Autodesk Fusion 360 part; units mm, degrees
sketch "Sketch1" plane through (0, 0, 0) normal (0, 0, 1) x (1, 0, 0)
  line L0 (0, 0) -> (69, 0)
  line L1 (69, 0) -> (69, 140)
  line L2 (69, 140) -> (0, 140)
  line L3 (0, 140) -> (0, 0)
  line L4 (0, 140) -> (-3, 140)
  line L5 (-3, 140) -> (-3, 0)
  line L6 (-3, 0) -> (0, 0)
  line L7 (0, 0) -> (0, 140)
  line L8 (69, 140) -> (72, 140)
  line L9 (72, 140) -> (72, 0)
  line L10 (72, 0) -> (69, 0)
  line L11 (69, 0) -> (69, 140)
  line L12 (34.5, 140) -> (34.5, 0) construction
  line L13 (25, 0) -> (44, 0)
  line L14 (44, 0) -> (44, 2)
  line L15 (44, 2) -> (25, 2)
  line L16 (25, 2) -> (25, 0)
  line L17 (34.5, 2) -> (34.5, 0) construction
  line L18 (53.1198, 29) -> (65.1198, 29)
  line L19 (65.1198, 29) -> (65.1198, 15)
  line L20 (65.1198, 15) -> (53.1198, 15)
  line L21 (53.1198, 15) -> (53.1198, 29)
  circle A0 centre (8, 75) radius 3.175
  circle A1 centre (61.6198, 40) radius 3.5
  line L22 (65.1198, 29) -> (65.1198, 49) construction
  dimension "d1" = 140
  dimension "d3" = 3
  dimension "d4" = 3
  dimension "d30" = 75
  dimension "d31" = 2
  dimension "d32" = 19
  dimension "d33" = 14
  dimension "d34" = 12
  dimension "d35" = 6.35
  dimension "d36" = 65
  dimension "d37" = 7
  dimension "d38" = 40
  dimension "d39" = 15
extrude "Extrude1" add sketch "Sketch1" along normal blind 3 contours L0 L1 L2 L3 L7 L11 L14 L15 L16
extrude "Extrude2" add sketch "Sketch1" along normal blind 40 contours L3 L4 L5 L6 L7 | L1 L8 L9 L10 L11
sketch "Sketch3" plane through (72, 0, 0) normal (1, 0, 0) x (0, 1, 0)
  line L0 (0, 0) -> (140, 0)
  line L1 (140, 0) -> (140, 40)
  line L2 (140, 40) -> (0, 40)
  line L3 (0, 40) -> (0, 0)
  line L4 (140, 0) -> (0, 0)
  line L5 (70, 40) -> (70, 0) construction
  line L6 (17.5, 40) -> (22.5, 40)
  line L7 (22.5, 40) -> (22.5, 37)
  line L8 (20.5, 35) -> (19.5, 35)
  line L9 (17.5, 37) -> (17.5, 40)
  arc A0 (17.5, 37) -> (19.5, 35) centre (19.5, 37) ccw
  arc A1 (20.5, 35) -> (22.5, 37) centre (20.5, 37) ccw
  line L10 (20, 40) -> (20, 35) construction
  line L11 (117.5, 40) -> (122.5, 40)
  line L12 (122.5, 40) -> (122.5, 37)
  line L13 (120.5, 35) -> (119.5, 35)
  line L14 (117.5, 37) -> (117.5, 40)
  arc A2 (117.5, 37) -> (119.5, 35) centre (119.5, 37) ccw
  arc A3 (120.5, 35) -> (122.5, 37) centre (120.5, 37) ccw
  line L15 (120, 35) -> (120, 40) construction
  point P0 (17.5, 35)
  point P1 (117.5, 35)
  dimension "d18" = 5
  dimension "d19" = 5
  dimension "d20" = 2
  dimension "d21" = 2
  dimension "d23" = 5
  dimension "d24" = 2
  dimension "d25" = 2
  dimension "d26" = 5
  dimension "d27" = 100
extrude "Extrude3" cut sketch "Sketch3" along normal mid plane 200 contours L2 L6 L7 L8 L9 A0 A1 | L2 L11 L12 L13 L14 A2 A3
Build history of the part. All positions in model axes, mm. A direction names the side the tool comes from. Round coordinates to 2 decimals unless told otherwise and drop trailing zeros. Loops run counter-clockwise (first coordinate to the right, second up) from the corner with the lowest first, then second, coordinate; pieces in that order, holes last.
Item 1: Saw through at A-A (x = 8). List the corners of the cut face in (y, z) (3 decimals), then the cut area to 3 significant figures.
Item 2: Saw through at D-D (y = 102.5). List the corners of the cut face in (x, z), then the cut area to 3 significant figures.
Item 3: Saw through at B-B (y = 40). List the corners of the cut face in (x, z), then the cut area to 3 significant figures.
Item 4: Two-plate mould, pull along Y, no slides. Class faces 5 (the face through (69.3, 0, 12.5)), 6 (the face through (7.59, 71.85, 1.48)), 7 (the face through (70, 131, 40)): released by +Y, released by -Y, zero draft, split by the parting line, or undercut.
Item 5: Pin check, flat tips, straight feed: P1, Ø0.5, axis at x = 70.5, y = 20, coming from the +Z side; P2, Ø1.5, axis at x = 18, y = 75.5, coming from the +Z side; P3, Ø2.5, axis at x = 33.5, z = 2, coming from the -Y side. Stop position of each tip, or through.
Item 6: Which spindle directions (+Z, -Z, +X, -X, +Y, -Y) get a long thin tool onto all of the face, cutting with end or side? Do faces 1 (the face through (53.12, 22, 1)), 2 (the face through (70, 17.5, 38)), 3 (the face through (34, 71, 3)), 4 (the face through (72, 71, 20)). Say none if no direction does.
Item 7: Drill centre lines: line 1 along X through (y, z) = (92, 31); line 2 along Y through (x, z) = (8, 1) (3 decimals); line 3 along Z through (x, y) = (58, 116.5). Where is each one in solid material? Low to high.
Item 8: Saw through at C-C (z = 22.5). List the corners of the cut face in (x, y), then the cut area to 3 significant figures.
Worked answers:
1. outline: (0, 0) - (71.825, 0) - (71.825, 3) - (0, 3) - close; (78.175, 0) - (140, 0) - (140, 3) - (78.175, 3) - close
1. area: 401 mm2
2. outline: (-3, 0) - (72, 0) - (72, 40) - (69, 40) - (69, 3) - (0, 3) - (0, 40) - (-3, 40) - close
2. area: 447 mm2
3. outline: (-3, 0) - (58.12, 0) - (58.12, 3) - (0, 3) - (0, 40) - (-3, 40) - close; (65.12, 0) - (72, 0) - (72, 40) - (69, 40) - (69, 3) - (65.12, 3) - close
3. area: 426 mm2
4. face 5: released by -Y
4. face 6: undercut
4. face 7: zero draft
5. P1: stops at z = 35
5. P2: stops at z = 3
5. P3: stops at y = 2
6. face 1: +Z, -Z
6. face 2: +Z, +X, -X
6. face 3: +Z, +Y, -Y
6. face 4: +Z, -Z, +X, +Y, -Y
7. line 1: x = -3 to 0, 69 to 72
7. line 2: y = 0 to 71.825, 78.175 to 140
7. line 3: z = 0 to 3
8. outline: (-3, 0) - (0, 0) - (0, 140) - (-3, 140) - close; (69, 0) - (72, 0) - (72, 140) - (69, 140) - close
8. area: 840 mm2
